```python
from build123d import *

# Parameters (mm, degrees)
BOX088_W           = 25
BOX088_H           = 24
BOX088_DEPTH       = 1.8
BOX088_PITCH_ANGLE = -90
BOX089_W           = 25
BOX089_H           = 21
BOX089_DEPTH       = 10
BOX089_PITCH_ANGLE = -90
CYLINDER297_R      = 1.45
CYLINDER297_DEPTH  = 2
BOX085_W           = 8
BOX085_H           = 6.4
BOX085_DEPTH       = 2
CYLINDER298_R      = 3.2
CYLINDER298_DEPTH  = 2
BOX086_W           = 4
BOX086_H           = 55.4
BOX086_DEPTH       = 26
CYLINDER295_R      = 1.45
CYLINDER295_DEPTH  = 2
BOX084_W           = 8
BOX084_H           = 6.4
BOX084_DEPTH       = 2
CYLINDER296_R      = 3.2
CYLINDER296_DEPTH  = 2
CHAMFER_SIZE       = 1
BOX087_W           = 14
BOX087_H           = 30
BOX087_DEPTH       = 5
BOX087_PITCH_ANGLE = -90
CHAMFER001_SIZE    = 8
FILLET_R           = 1
FILLET001_R        = 1
CHAMFER002_SIZE    = 1
CHAMFER003_SIZE    = 1
CHAMFER004_SIZE    = 0.45


with BuildPart() as cubo088:
    # Box088 → Box088 (new body)
    with BuildSketch(Plane.XY):
        with Locations((12.5, 12)):
            Rectangle(BOX088_W, BOX088_H)
    extrude(amount=BOX088_DEPTH)


with BuildPart() as cubo088_1:
    # Box088 pitch: moved
    add(cubo088.part.rotate(Axis((0, 0, 0), (0, 1, 0)), BOX088_PITCH_ANGLE))


with BuildPart() as cubo088_2:
    # Box088 placement: moved
    add(cubo088_1.part.moved(Location((-44, -10.2, 76))))


with BuildPart() as fusion128:
    # Box089 → Box089 (new body)
    with BuildSketch(Plane.XY):
        with Locations((12.5, 10.5)):
            Rectangle(BOX089_W, BOX089_H)
    extrude(amount=BOX089_DEPTH)


with BuildPart() as fusion128_1:
    # Box089 pitch: moved
    add(fusion128.part.rotate(Axis((0, 0, 0), (0, 1, 0)), BOX089_PITCH_ANGLE))


with BuildPart() as fusion128_2:
    # Box089 placement: moved
    add(fusion128_1.part.moved(Location((-41, -8.7, 76))))

    # Fusion128: union Cubo088
    add(cubo088_2.part)


with BuildPart() as fusion128_3:
    # Fusion128 placement: moved
    add(fusion128_2.part.moved(Location((-0.5, -0.7, 0))))


with BuildPart() as cilindro297:
    # Cylinder297 → Cylinder297 (new body)
    with BuildSketch(Plane.XY):
        Circle(CYLINDER297_R)
    extrude(amount=CYLINDER297_DEPTH)


with BuildPart() as cubo085:
    # Box085 → Box085 (new body)
    with BuildSketch(Plane(origin=(-8, -3.2, 0), x_dir=(1, 0, 0), z_dir=(0, 0, 1))):
        with Locations((4, 3.2)):
            Rectangle(BOX085_W, BOX085_H)
    extrude(amount=BOX085_DEPTH)


with BuildPart() as cut009:
    # Cylinder298 → Cylinder298 (new body)
    with BuildSketch(Plane.XY):
        Circle(CYLINDER298_R)
    extrude(amount=CYLINDER298_DEPTH)

    # Fusion126: union Cubo085
    add(cubo085.part)

    # Cut009: cut Cilindro297
    add(cilindro297.part, mode=Mode.SUBTRACT)


with BuildPart() as cut009_1:
    # Cut009 placement: moved
    add(cut009.part.moved(Location((-39.5, 25.5, 61.6))))


with BuildPart() as cubo086:
    # Box086 → Box086 (new body)
    with BuildSketch(Plane(origin=(-47.5, -26.7, 61.6), x_dir=(1, 0, 0), z_dir=(0, 0, 1))):
        with Locations((2, 27.7)):
            Rectangle(BOX086_W, BOX086_H)
    extrude(amount=BOX086_DEPTH)


with BuildPart() as cilindro295:
    # Cylinder295 → Cylinder295 (new body)
    with BuildSketch(Plane.XY):
        Circle(CYLINDER295_R)
    extrude(amount=CYLINDER295_DEPTH)


with BuildPart() as cubo084:
    # Box084 → Box084 (new body)
    with BuildSketch(Plane(origin=(-8, -3.2, 0), x_dir=(1, 0, 0), z_dir=(0, 0, 1))):
        with Locations((4, 3.2)):
            Rectangle(BOX084_W, BOX084_H)
    extrude(amount=BOX084_DEPTH)


with BuildPart() as chamfer_body:
    # Cylinder296 → Cylinder296 (new body)
    with BuildSketch(Plane.XY):
        Circle(CYLINDER296_R)
    extrude(amount=CYLINDER296_DEPTH)

    # Fusion125: union Cubo084
    add(cubo084.part)

    # Cut008: cut Cilindro295
    add(cilindro295.part, mode=Mode.SUBTRACT)


with BuildPart() as chamfer_body_1:
    # Cut008 placement: moved
    add(chamfer_body.part.moved(Location((-39.5, -23.5, 61.6))))

    # Fusion127: union Cut009, Cubo086
    add(cut009_1.part)
    add(cubo086.part)

    # Chamfer
    chamfer_edges = [chamfer_body_1.edges().sort_by_distance(p)[0] for p in [
        (-43.5, 25.5, 63.6),
        (-43.5, -23.5, 63.6),
    ]]
    chamfer(chamfer_edges, length=CHAMFER_SIZE)


with BuildPart() as chamfer004:
    # Box087 → Box087 (new body)
    with BuildSketch(Plane.XY):
        with Locations((7, 15)):
            Rectangle(BOX087_W, BOX087_H)
    extrude(amount=BOX087_DEPTH)


with BuildPart() as chamfer004_1:
    # Box087 pitch: moved
    add(chamfer004.part.rotate(Axis((0, 0, 0), (0, 1, 0)), BOX087_PITCH_ANGLE))


with BuildPart() as chamfer004_2:
    # Box087 placement: moved
    add(chamfer004_1.part.moved(Location((-43, -14, 76))))

    # Fusion129: union Chamfer body
    add(chamfer_body_1.part)

    # Cut010: cut Fusion128
    add(fusion128_3.part, mode=Mode.SUBTRACT)

    # Chamfer001
    chamfer001_edges = [chamfer004_2.edges().sort_by_distance(p)[0] for p in [
        (-45.5, -26.7, 87.6),
        (-45.5, 28.7, 87.6),
    ]]
    chamfer(chamfer001_edges, length=CHAMFER001_SIZE)

    # Fillet
    fillet_edges = [chamfer004_2.edges().sort_by_distance(p)[0] for p in [
        (-45.5, -26.7, 79.6),
        (-45.5, -18.7, 87.6),
        (-45.5, 20.7, 87.6),
        (-45.5, 28.7, 79.6),
    ]]
    fillet(fillet_edges, radius=FILLET_R)

    # Fillet001
    fillet001_edges = [chamfer004_2.edges().sort_by_distance(p)[0] for p in [
        (-45.5, -14, 87.6),
        (-45.5, 16, 87.6),
    ]]
    fillet(fillet001_edges, radius=FILLET001_R)

    # Chamfer002
    chamfer002_edges = [chamfer004_2.edges().sort_by_distance(p)[0] for p in [
        (-45.4, -10.9, 90),
        (-45.4, 13.1, 90),
    ]]
    chamfer(chamfer002_edges, length=CHAMFER002_SIZE)

    # Chamfer003
    chamfer003_edges = [chamfer004_2.edges().sort_by_distance(p)[0] for p in [
        (-44.5, -10.15, 90),
        (-46.3, -10.15, 90),
        (-44.5, 12.35, 90),
        (-46.3, 12.35, 90),
    ]]
    chamfer(chamfer003_edges, length=CHAMFER003_SIZE)

    # Chamfer004
    chamfer004_edges = [chamfer004_2.edges().sort_by_distance(p)[0] for p in [
        (-43.5, -11.7, 76),
        (-47.5, -11.7, 76),
        (-47.5, 13.8, 76),
        (-43.5, 13.8, 76),
    ]]
    chamfer(chamfer004_edges, length=CHAMFER004_SIZE)


solid = chamfer004_2.part
```
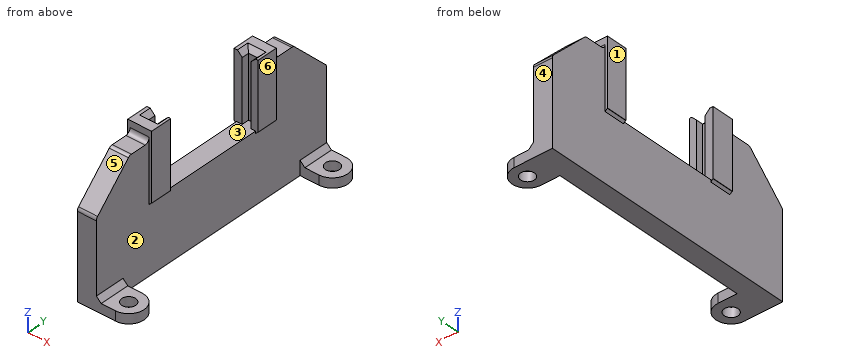
Check sheet for the modelled part. Datum: model origin and axes. Units: mm. Face numbers are marked on the shaded views. A direction names the side the tool comes from. Round coordinates to 2 decimals unless told otherwise and drop trailing zeros. Order: outer loops, then holes, each group sorted by start corner. A loop starts at its lowest first (then second) coordinate and runs counter-clockwise, first axis right, second up.
1) Section check B-B (x = -41.75). Record the boundary of the cut face in (y, z), and give its area (3 significant figures).
2) Section check D-D (z = 86.5). Record the boundary of the cut face in (x, y), and give its area (3 significant figures).
3) Scan lines: line 1 (Y direction, x = -39.5, z = 62.3); line 2 (X direction, y = 14, z = 85.75); line 3 (X direction, y = 11, z = 64). Record each from-to range of solid material in increasing order.
4) Go/stop test with flat-tipped pins: pin 1 Ø2 at (x, z) = (-45.5, 82.5) entering from +Y; pin 2 Ø5 at (y, z) = (2.5, 77) entering from -X; pin 3 Ø6 at (y, z) = (-6.5, 76) entering from +X. Record where each tip stops, or that it passes through.
5) Section check A-A (y = -23.5). Record the boundary of the cut face in (x, z).
6) Mould release check, pull along Y, two halves, no side actions. Record for the marked faces 3, 4, 5 and 6: +Y half, -Y half, draft (parallel to the pull), parting line (faces both ways), or undercut.
7) Tool access check on the marked faces 1 and 2. Record the directions out of +Z, -Z, +X, -X, +Y, -Y that give a thin tool (end or side, any length) a straight path to the whole face; none if there is none.
8) Section check C-C (z = 83.25). Record the boundary of the cut face in (x, y).
Result:
1. outline: (-26.7, 61.6) - (-20.3, 61.6) - (-20.3, 63.6) - (-26.7, 63.6) - close; (22.3, 61.6) - (28.7, 61.6) - (28.7, 63.6) - (22.3, 63.6) - close
1. area: 25.6 mm2
2. outline: (-48, -14) - (-47.5, -14) - (-47.5, -19.8) - (-43.5, -19.8) - (-43.5, -14) - (-43, -14) - (-43, -9.4) - (-44.5, -9.4) - (-44.5, -10.9) - (-46.3, -10.9) - (-46.3, -9.4) - (-48, -9.4) - close; (-48, 11.6) - (-46.3, 11.6) - (-46.3, 13.1) - (-44.5, 13.1) - (-44.5, 11.6) - (-43, 11.6) - (-43, 16) - (-43.5, 16) - (-43.5, 21.8) - (-47.5, 21.8) - (-47.5, 16) - (-48, 16) - close
2. area: 86.0 mm2
3. line 1: y = -26.7 to -24.95, -22.05 to -20.3, 22.3 to 24.05, 26.95 to 28.7
3. line 2: x = -48 to -43
3. line 3: x = -47.5 to -43.5
4. pin 1: stops at y = 26.8
4. pin 2: stops at x = -47.5
4. pin 3: stops at x = -43
5. outline: (-47.5, 61.6) - (-40.95, 61.6) - (-40.95, 63.6) - (-42.5, 63.6) - (-43.5, 64.6) - (-43.5, 82.8) - (-47.5, 82.8) - close; (-38.05, 61.6) - (-36.3, 61.6) - (-36.3, 63.6) - (-38.05, 63.6) - close
6. face 3: undercut
6. face 4: +Y half
6. face 5: -Y half
6. face 6: draft
7. face 1: +Z, -Z, -X, +Y, -Y
7. face 2: +X
8. outline: (-48, -14) - (-47.5, -14) - (-47.5, -23.05) - (-43.5, -23.05) - (-43.5, -14) - (-43, -14) - (-43, -9.4) - (-44.5, -9.4) - (-44.5, -10.9) - (-46.3, -10.9) - (-46.3, -9.4) - (-48, -9.4) - close; (-48, 11.6) - (-46.3, 11.6) - (-46.3, 13.1) - (-44.5, 13.1) - (-44.5, 11.6) - (-43, 11.6) - (-43, 16) - (-43.5, 16) - (-43.5, 25.05) - (-47.5, 25.05) - (-47.5, 16) - (-48, 16) - close
